Part print with two shaded views. Sizes in mm from the minimum x, y, z corner. Round coordinates to 2 decimals unless told otherwise and drop trailing zeros. Write each loop counter-clockwise with the first axis right and the second up, starting at its lowest first coordinate (ties: lowest second). Pieces come first, ordered by that corner, then holes. Notation, with made-up numbers: M -38.5,16 L -7.5,16 A27 cw -7.5,37 Z; hole C -14,30 d3. An arc over 180 degrees is marked long. Use one line per item in the form item = value. Start each with the question number.
Item 1: Mould opens along Y. For the marked faces 1, 2, 3 and 4 say: +Y half, -Y half, draft (parallel to the pull), parting line (faces both ways), or undercut.
Item 2: Cut at D-D, the plane y = 31. Give the cut face in (x, z).
Item 3: Cut at B-B, the plane y = 15. Give the cut face in (x, z), then the cut area to 3 significant figures.
Item 4: Probe L1, parallel to X at y = 15, z = 44; L2, parallel to X at y = 26.5, z = 46.5; L3, parallel to Y at x = 23.5, z = 73. List the from-to ranges inside material, lowest first.
Item 5: Cut at A-A, the plane x = 15. Give the cut face in (y, z).
Item 6: Flat gauge pins, fed straight in: pin 1 Ø3 at (y, z) = (31, 51) entering from +X; pin 2 Ø3 at (y, z) = (31, 47) entering from -X; pin 3 Ø4 at (y, z) = (20, 43) entering from -X. Where does each tip first touch, or does it go through?
Item 7: Cut at C-C, the plane z = 5. Give the cut face in (x, y), then the cut area to 3 significant figures.
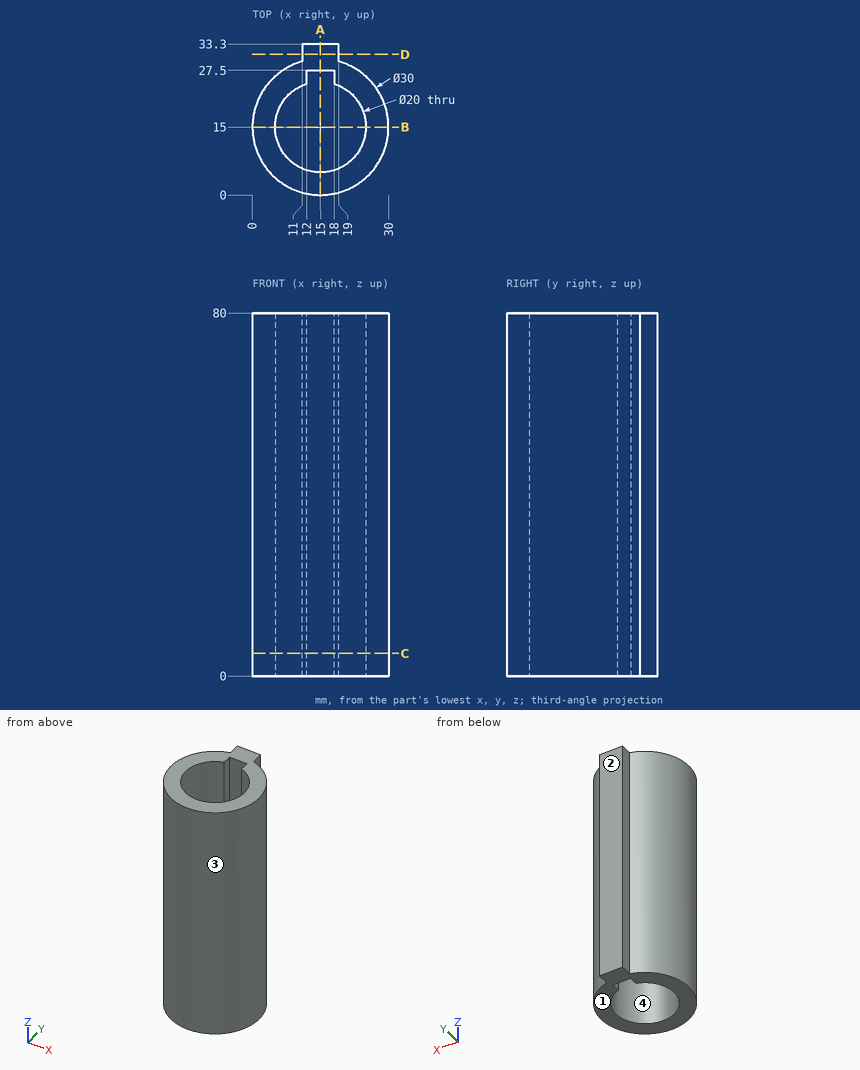
Model answer:
q1.face_1 = draft
q1.face_2 = +Y half
q1.face_3 = parting line
q1.face_4 = undercut
q2.outline = M 11,0 L 19,0 L 19,80 L 11,80 Z
q3.outline = M 0,0 L 5,0 L 5,80 L 0,80 Z; M 25,0 L 30,0 L 30,80 L 25,80 Z
q3.area = 800 mm²
q4.L1 = 0 to 5, 25 to 30
q4.L2 = 5.37 to 12, 18 to 24.63
q4.L3 = 2.64 to 9.73, 20.27 to 27.36
q5.outline = M 0,0 L 5,0 L 5,80 L 0,80 Z; M 27.5,0 L 33.3,0 L 33.3,80 L 27.5,80 Z
q6.pin_1 = 19
q6.pin_2 = 11
q6.pin_3 = 0.3
q7.outline = M 11,29.46 A15 ccw long 19,29.46 L 19,33.3 L 11,33.3 Z; hole M 12,24.54 A10 ccw long 18,24.54 L 18,27.5 L 12,27.5 Z
q7.area = 405 mm²
